```python
from build123d import *

# Parameters (mm, degrees)
BOSS_EXTRUDE1_DEPTH = 5.842
FILLET1_R           = 1.5875


with BuildPart() as part:
    # Sketch1 → Boss-Extrude1 (new body)
    with BuildSketch(Plane.XY):
        Polygon((50.8, -22.225), (44.45, -22.225), (44.45, -19.05), (-44.45, -19.05), (-44.45, -22.225), (-50.8, -22.225), (-50.8, -19.05), (-56.642, -19.05), (-56.642, -6.35), (-50.8, -6.35), (-50.8, 6.35), (-56.642, 6.35), (-56.642, 19.05), (-50.8, 19.05), (-50.8, 31.75), (-56.642, 31.75), (-56.642, 44.45), (-50.8, 44.45), (-50.8, 47.498), (50.8, 47.498), (50.8, 44.45), (56.642, 44.45), (56.642, 31.75), (50.8, 31.75), (50.8, 19.05), (56.642, 19.05), (56.642, 6.35), (50.8, 6.35), (50.8, -6.35), (56.642, -6.35), (56.642, -19.05), (50.8, -19.05), align=None)
    extrude(amount=BOSS_EXTRUDE1_DEPTH)

    # Fillet1
    fillet1_edges = [part.edges().sort_by_distance(p)[0] for p in [
        (-44.45, -19.05, 2.921),
        (44.45, -19.05, 2.921),
    ]]
    fillet(fillet1_edges, radius=FILLET1_R)
    fillet1_2_edges = [part.edges().sort_by_distance(p)[0] for p in [
        (44.45, -22.225, 2.921),
        (-44.45, -22.225, 2.921),
    ]]
    fillet(fillet1_2_edges, radius=FILLET1_R - 0.0001)  # a hair under: the kernel refuses the full size


solid = part.part
```
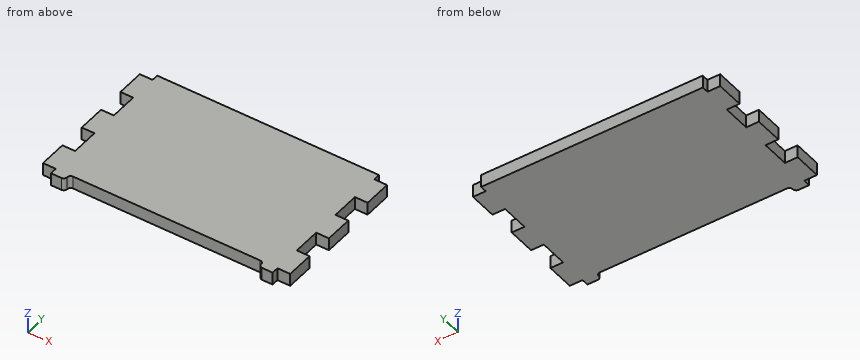
Verification items for the finished model (mm, model axes). Round coordinates to 2 decimals unless told otherwise and drop trailing zeros. Order: outer loops, then holes, each group sorted by start corner. A loop starts at its lowest first (then second) coordinate and runs counter-clockwise, first axis right, second up. Notation, with made-up numbers: (-20.5, -39) - (38.5, -39) arc R4 cw to (38.5, -35) - close; hole circle Ø5 at (-32, -16). An arc over 180 degrees is marked (long way). Use CSV: the item, a comma, the result in double quotes.
(1) Gauge pin test, flat ends, axial feed: pin 1 Ø8 at (x, y) = (31, 23.5) entering from -Z; pin 2 Ø3 at (x, z) = (-54.5, 3.5) entering from -Y; pin 3 Ø1 at (y, z) = (-5, 2.5) entering from +X; pin 4 Ø3 at (x, z) = (55, 1.5) entering from +Y. Record the tip position at first contact, or that the pin passes through.
Entries:
pin 1,"z = 0"
pin 2,"y = -19.05"
pin 3,"x = 50.8"
pin 4,"y = 44.45"
(2) Section check B-B on y = 29. Record the boundary of the cut face in (x, z), and give its area (3 significant figures).
Entries:
outline,"(-50.8, 0) - (50.8, 0) - (50.8, 5.84) - (-50.8, 5.84) - close"
area,"594 mm^2"
(3) Thickness scan on probe 1 along Y at (x, z) = (-30, 0.7); probe 2 along X at (y, z) = (-1, 1.25). Record the ranges inside material, lowest first. Write a range as from..to.
Entries:
probe 1,"-19.05..47.5"
probe 2,"-50.8..50.8"
(4) Section check A-A on x = 11. Record the boundary of the cut face in (y, z), and give its area (3 significant figures).
Entries:
outline,"(-19.05, 0) - (47.5, 0) - (47.5, 5.84) - (-19.05, 5.84) - close"
area,"389 mm^2"
